```python
from build123d import *

# Parameters (mm, degrees)
SKETCH1_W              = 44.45
SKETCH1_H              = 25.4
BOSS_EXTRUDE1_DEPTH    = 25.4
F_10_CLEARANCE_HOLE1_D = 5.1054
CHAMFER1_SIZE          = 3.175


with BuildPart() as part:
    # Sketch1 → Boss-Extrude1 (new body)
    with BuildSketch(Plane(origin=(0, 0, 0), x_dir=(1, 0, 0), z_dir=(0, 1, 0))):
        Rectangle(SKETCH1_W, SKETCH1_H)
    extrude(amount=BOSS_EXTRUDE1_DEPTH)

    # #10 Clearance Hole1 (through all)
    with Locations(Plane(origin=(0, 25.4, 0), x_dir=(1, 0, 0), z_dir=(0, 1, 0))):
        with Locations((-15.875, 0), (15.875, 0)):
            Hole(F_10_CLEARANCE_HOLE1_D / 2)

    # Chamfer1
    chamfer1_edges = [part.edges().sort_by_distance(p)[0] for p in [
        (22.225, 12.7, 12.7),
        (-22.225, 12.7, 12.7),
        (-22.225, 12.7, -12.7),
        (22.225, 12.7, -12.7),
    ]]
    chamfer(chamfer1_edges, length=CHAMFER1_SIZE)


solid = part.part
```
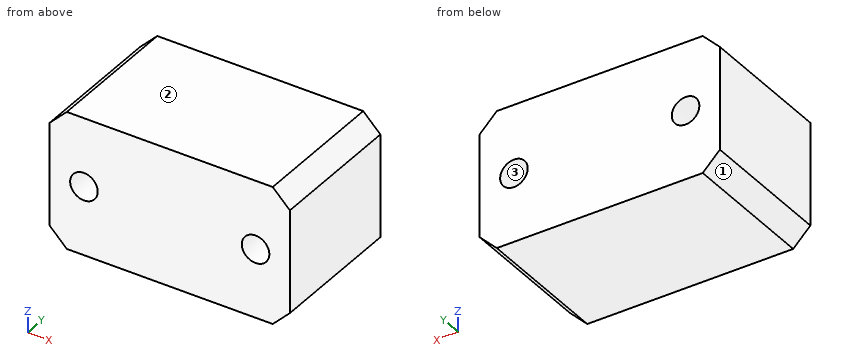
Geometry check sheet. Reference: the model listing, model coordinates, mm. Face numbers are marked on the shaded views. Coordinates: 2 decimals unless noted, no trailing zeros. Order: outer loops, then holes, each group sorted by start corner. A loop starts at its lowest first (then second) coordinate and runs counter-clockwise, first axis right, second up.
Item 1: Scan lines: line 1 along Z through (x, y) = (-16, 6); line 2 along X through (y, z) = (12.5, -2) (3 decimals); line 3 along Z through (x, y) = (18, 7.25). Record each from-to range of solid material in increasing order.
Item 2: Section check C-C (x = 16.5). Enter the section's corners in (y, z) (3 decimals), plus the area to 3 significant figures.
Item 3: Depth check by flat-ended pin: pin 1 (4 mm diameter, centred on x = -15.875, z = 0, fed in from +Y). Enter the tip coordinate at first touch or a pass-through.
Item 4: Mould release check, pull along Z, two halves, no side actions. Record for the marked faces 1, 2 and 3: released by +Z, released by -Z, zero draft, split by the parting line, or undercut.
Item 5: Section check B-B (y = 23.75). Enter the section's corners in (x, z) (3 decimals).
Item 6: Section check A-A (z = 0). Enter the section's corners in (x, y) (3 decimals).
Item 7: Section check D-D (x = -17.5). Enter the section's corners in (y, z).
Check sheet entries:
1. line 1: z = -12.7 to -2.55, 2.55 to 12.7
1. line 2: x = -22.225 to -17.461, -14.289 to 14.289, 17.461 to 22.225
1. line 3: z = -12.7 to -1.41, 1.41 to 12.7
2. outline: (0, -12.7) - (25.4, -12.7) - (25.4, -2.475) - (0, -2.475) - close; (0, 2.475) - (25.4, 2.475) - (25.4, 12.7) - (0, 12.7) - close
2. area: 519 mm2
3. pin 1: passes through
4. face 1: released by -Z
4. face 2: released by +Z
4. face 3: undercut
5. outline: (-22.225, -9.525) - (-19.05, -12.7) - (19.05, -12.7) - (22.225, -9.525) - (22.225, 9.525) - (19.05, 12.7) - (-19.05, 12.7) - (-22.225, 9.525) - close; hole circle Ø5.105 at (-15.875, 0); hole circle Ø5.105 at (15.875, 0)
6. outline: (-22.225, 0) - (-18.428, 0) - (-18.428, 25.4) - (-22.225, 25.4) - close; (-13.322, 0) - (13.322, 0) - (13.322, 25.4) - (-13.322, 25.4) - close; (18.428, 0) - (22.225, 0) - (22.225, 25.4) - (18.428, 25.4) - close
7. outline: (0, -12.7) - (25.4, -12.7) - (25.4, -1.97) - (0, -1.97) - close; (0, 1.97) - (25.4, 1.97) - (25.4, 12.7) - (0, 12.7) - close
